Autodesk Inventor part; units mm, degrees
ref_plane "YZ Plane" through (0, 0, 0) normal (1, 0, 0) x (0, 1, 0)
ref_plane "XZ Plane" through (0, 0, 0) normal (0, 1, 0) x (-1, 0, 0)
ref_plane "XY Plane" through (0, 0, 0) normal (0, 0, 1) x (1, 0, 0)
sketch "Sketch1" plane through (0, 0, 0) normal (0, 0, 1) x (1, 0, 0)
  line L0 (-40, 87.5) -> (40, 87.5)
  line L1 (40, 87.5) -> (40, -87.5)
  line L2 (40, -87.5) -> (-40, -87.5)
  line L3 (-40, -87.5) -> (-40, 87.5)
  point P0 (0, 0)
  dimension "d0" = 80
  dimension "d1" = 175
  dimension "d2" = 40
  dimension "d3" = 87.5
extrude "Extrusion1" add sketch "Sketch1" along normal blind 3.4163
sketch "Sketch2" plane through (0, 0, 3.4163) normal (0, 0, 1) x (1, 0, 0)
  line L0 (40, 87.5) -> (-40, 87.5)
  line L1 (-40, 87.5) -> (-40, -87.5)
  circle A0 centre (-32.3, 77.3) radius 2.75
  circle A1 centre (32.3, 77.3) radius 2.75
  point P0 (0, 0)
  dimension "d6" = 5.5
  dimension "d7" = 10.2
  dimension "d12" = 5.5
  dimension "d13" = 64.6
  dimension "d14" = 7.7
  dimension "d15" = 10.2
extrude "Extrusion2" cut sketch "Sketch2" against normal through all
pattern_linear "Rectangular Pattern1" count 2 spacing 154.6 along (0, -1, 0) of "Extrusion2"
sketch "Sketch3" plane through (0, 0, 3.4163) normal (0, 0, 1) x (1, 0, 0)
  line L0 (40, 87.5) -> (-40, 87.5)
  line L1 (-40, 87.5) -> (-40, -87.5)
  line L2 (-30, 11) -> (-30, -11) construction
  line L3 (-32.75, 11) -> (-32.75, -11)
  line L4 (-27.25, -11) -> (-27.25, 11)
  arc A0 (-27.25, 11) -> (-32.75, 11) centre (-30, 11) ccw
  arc A1 (-32.75, -11) -> (-27.25, -11) centre (-30, -11) ccw
  point P0 (0, 0)
  point P1 (-30, 0)
  dimension "d25" = 22
  dimension "d26" = 5.5
  dimension "d27" = 76.5
  dimension "d35" = 10
extrude "Extrusion3" cut sketch "Sketch3" against normal through all
sketch "Sketch4" plane through (0, 0, 3.4163) normal (0, 0, 1) x (1, 0, 0)
  circle A0 centre (-32.3, -77.3) radius 2.75
  circle A1 centre (32.3, -77.3) radius 2.75
  circle A2 centre (-32.3, -77.3) radius 3.58
  circle A3 centre (32.3, -77.3) radius 3.58
  point P0 (0, 0)
  dimension "d31" = 7.16
  dimension "d32" = 7.16
extrude "Extrusion4" cut sketch "Sketch4" against normal through all
fillet "Fillet1" radius 2 4 edges at (40, 87.5, 1.7082) (-40, 87.5, 1.7082) (-40, -87.5, 1.7082) (40, -87.5, 1.7082)
sketch "Sketch5" plane through (0, 0, 3.4163) normal (0, 0, 1) x (1, 0, 0)
  line L0 (38, 87.5) -> (-38, 87.5)
  line L1 (-40, 85.5) -> (-40, -85.5)
  circle A0 centre (-10, 77.5) radius 2.75
  line L2 (-38, -87.5) -> (38, -87.5)
  circle A1 centre (-10, 10) radius 2.75
  circle A2 centre (-10, -10) radius 2.75
  circle A3 centre (-10, -77.5) radius 2.75
  point P0 (0, 0)
  dimension "d37" = 5.5
  dimension "d38" = 30
  dimension "d39" = 10
  dimension "d48" = 5.5
  dimension "d49" = 77.5
  dimension "d50" = 5.5
  dimension "d51" = 97.5
  dimension "d52" = 5.5
  dimension "d53" = 10
  dimension "d54" = 30
  dimension "d55" = 30
  dimension "d56" = 30
extrude "Extrusion5" cut sketch "Sketch5" against normal through all
pattern_linear "Rectangular Pattern3" count 2 spacing 20 along (1, 0, 0) of "Extrusion5"
equation "\"d15\" = d7"
properties part number "x-carriage" material "Steel, Mild"
For this review, take the finished solid that the model builds, in its own axes (mm). A direction names the side the tool comes from. Coordinates: 2 decimals unless noted, no trailing zeros. Order: outer loops, then holes, each group sorted by start corner. A loop starts at its lowest first (then second) coordinate and runs counter-clockwise, first axis right, second up. Notation, with made-up numbers: (71, -30) - (120, -30) arc R21 cw to (120, -26) - close; hole circle Ø4 at (87, 66). An arc over 180 degrees is marked (long way). Answer as a JSON object with one key per item and string values. Group by question number.
1. We need section B-B on x = -11. State the section outline as (y, z) points.
2. We need section A-A on z = 1.15. Give the number of separate pieces and of enclosed holes in the cut face, then the cut area to 3 significant figures.
3. Clearance check with a flat-ended pin moving along its axis: P1, Ø11.5, axis at x = -32.3, y = -77.3, coming from the -Z side. State where the tip first meets the part, or that it passes through.
4. The part is to be moulded in two halves that separate along Y. For faces 3 (the flat face through (-1, 87.5, 2)), 4 (the cylindrical face through (-8.52, 79.82, 1.73)), 5 (the flat face through (-1, 1, 3.416)), say which applies: pulls with the +Y half, pulls with the -Y half, needs draft (parallel to the pull), parting line crosses it, or undercut.
5. For probe 1 along Y at (x, z) = (32.5, 0.55); probe 2 along Y at (x, z) = (-10, 2.75); probe 3 along Y at (x, z) = (-7.5, 2.2), list the stretches that pass through material, from the lowest coordinate up.
6. For faces 1 (the flat face through (-1, 1, 0)), 2 (the flat face through (-27.25, 0, 2)), list the 3-axis set-ups (+Z, -Z, +X, -X, +Y, -Y) from which the entire face can be reached by the end or side of a thin tool; tool diameter is ignored.
Final values:
{
 "1": {"outline": "(-87.5, 0) - (-80.06, 0) - (-80.06, 3.42) - (-87.5, 3.42) - close; (-74.94, 0) - (-12.56, 0) - (-12.56, 3.42) - (-74.94, 3.42) - close; (-7.44, 0) - (7.44, 0) - (7.44, 3.42) - (-7.44, 3.42) - close; (12.56, 0) - (74.94, 0) - (74.94, 3.42) - (12.56, 3.42) - close; (80.06, 0) - (87.5, 0) - (87.5, 3.42) - (80.06, 3.42) - close"},
 "2": {"separate pieces": "1", "enclosed holes": "13", "area": "13,500 mm²"},
 "3": {"P1": "z = 0"},
 "4": {"face 3": "pulls with the +Y half", "face 4": "undercut", "face 5": "needs draft"},
 "5": {"probe 1": "-87.5 to -80.87, -73.73 to 74.56, 80.04 to 87.5", "probe 2": "-87.5 to -80.25, -74.75 to -12.75, -7.25 to 7.25, 12.75 to 74.75, 80.25 to 87.5", "probe 3": "-87.5 to -78.65, -76.35 to -11.15, -8.85 to 8.85, 11.15 to 76.35, 78.65 to 87.5"},
 "6": {"face 1": "-Z, +X, -X, +Y, -Y", "face 2": "+Z, -Z"}
}
